from build123d import *

# Parameters (mm, degrees)
SKETCH_1_W             = 31
SKETCH_1_H             = 48
EXTRUDE_1_DEPTH        = 1.2
SKETCH_2_W             = 30.07
SKETCH_2_H             = 37.43
EXTRUDE_2_DEPTH        = 1.56
SKETCH_4_R             = 0.635
CUT_EXTRUDE_1_DEPTH    = 58.16146954
PATTERN_LINEAR_1_COUNT = 8
PATTERN_LINEAR_1_PITCH = 2.54
SKETCH_6_R             = 1
SKETCH_6_W             = 20
SKETCH_6_H             = 5.29
CUT_EXTRUDE_2_DEPTH    = 58.16146954


with BuildPart() as part:
    # 草图1 → 凸台-拉伸1 (new body)
    with BuildSketch(Plane(origin=(0, 0, 0), x_dir=(1, 0, 0), z_dir=(0, 1, 0))):
        with Locations((15.5, 24)):
            Rectangle(SKETCH_1_W, SKETCH_1_H)
    extrude(amount=EXTRUDE_1_DEPTH)

    # 草图2 → 凸台-拉伸2 (add)
    with BuildSketch(Plane(origin=(0, 1.2, 0), x_dir=(1, 0, 0), z_dir=(0, 1, 0))):
        with Locations((15.5, 24.005)):
            Rectangle(SKETCH_2_W, SKETCH_2_H)
    extrude(amount=EXTRUDE_2_DEPTH)

    # 草图4 → 切除-拉伸1 (cut, through all)
    with BuildSketch(Plane(origin=(0, 1.2, 0), x_dir=(1, 0, 0), z_dir=(0, 1, 0))):
        with Locations(Location((6.61, 46.5, 0), (0, 0, 270))):
            Circle(SKETCH_4_R)
    cut_extrude_1 = extrude(amount=-CUT_EXTRUDE_1_DEPTH, mode=Mode.SUBTRACT)

    # 阵列(线性)1: 切除-拉伸1 ×8
    with Locations(*[(i * PATTERN_LINEAR_1_PITCH, 0, 0) for i in range(1, PATTERN_LINEAR_1_COUNT)]):
        add(cut_extrude_1, mode=Mode.SUBTRACT)

    # 草图6 → 切除-拉伸2 (cut, through all)
    with BuildSketch(Plane(origin=(0, 1.2, 0), x_dir=(1, 0, 0), z_dir=(0, 1, 0))):
        with Locations(Location((2.5, 45.5, 0), (0, 0, 270))):
            Circle(SKETCH_6_R)
        with Locations(Location((28.5, 45.5, 0), (0, 0, 270))):
            Circle(SKETCH_6_R)
        with Locations(Location((2.5, 2.5, 0), (0, 0, 270))):
            Circle(SKETCH_6_R)
        with Locations(Location((28.5, 2.5, 0), (0, 0, 270))):
            Circle(SKETCH_6_R)
        with Locations((15.5, 2.645)):
            Rectangle(SKETCH_6_W, SKETCH_6_H)
    extrude(amount=-CUT_EXTRUDE_2_DEPTH, mode=Mode.SUBTRACT)


solid = part.part
The model under review builds one solid part; all positions refer to its coordinate system, in mm. A direction names the side the tool comes from. Round coordinates to 2 decimals unless told otherwise and drop trailing zeros. Write each loop counter-clockwise with the first axis right and the second up, starting at its lowest first coordinate (ties: lowest second). Pieces come first, ordered by that corner, then holes. Notation, with made-up numbers: M 41,71.25 L 52,71.25 A7 cw 52,79.25 Z; hole C -10,-30.75 d11. An arc over 180 degrees is marked long. Use a Markdown table: item, result. Add a question column.
Q1. Machinability: for faces 4 (the face through (15, 2, -42.72)), 5 (the face through (29.49, 0.61, -2.63)), 6 (the face through (25.5, 1, -3)), which of the approach directions +Z, -Z, +X, -X, +Y, -Y give a long, thin tool a straight path to every point of the face, cutting with its end or side? Answer none if there is none.
Q2. Insertion check: pin 1 (0.8 mm diameter, centred on y = 2, z = -31.5, fed in from +X) (3 decimals); pin 2 (1.5 mm diameter, centred on x = 24.39, z = -46.5, fed in from +Y). Each pin has a flat end and moves straight along its axis. Give the tip position at first contact, or say it passes through.
Q3. We need section C-C, the plane x = 2.5. State the section outline as (y, z) points, plus the area to 3 significant figures.
Q4. To check wall thickness, follow line 1 (X direction, y = 0.6, z = -2.5); line 2 (X direction, y = 1.15, z = -3); line 3 (X direction, y = 2, z = -7.5) (3 decimals). State the ranges of each line that lie inside material, in increasing order.
Q5. We need section B-B, the plane y = 0.75. Count the separate pieces of the cut face and the enclosed holes in it, plus the area to 3 significant figures.
Q6. We need section A-A, the plane z = -2.5. State the section outline as (x, y) points, plus the area to 3 significant figures.
Q7. We need section D-D, the plane x = 21.85. State the section outline as (y, z) points (3 decimals), plus the area to 3 significant figures.
Q8. The part is to be moulded in two halves that separate along X. For faces 1 (the face through (3, 1, 0)), 2 (the face through (0, 1, -24)), 3 (the face through (22.041, 0.608, -45.894)), say which applies: pulls with the +X half, pulls with the -X half, needs draft (parallel to the pull), parting line crosses it, or undercut.
Findings below:
| question | item | result |
|---|---|---|
| 1 | face 4 | -Z, +X, -X, +Y |
| 1 | face 5 | +Y, -Y |
| 1 | face 6 | +Z, +Y, -Y |
| 2 | pin 1 | stops at x = 30.535 |
| 2 | pin 2 | stops at y = 1.2 |
| 3 | outline | M 0,-48 L 1.2,-48 L 1.2,-46.5 L 0,-46.5 Z; M 0,-44.5 L 1.2,-44.5 L 1.2,-42.72 L 2.76,-42.72 L 2.76,-5.29 L 1.2,-5.29 L 1.2,-3.5 L 0,-3.5 Z; M 0,-1.5 L 1.2,-1.5 L 1.2,0 L 0,0 Z |
| 3 | area | 111 mm² |
| 4 | line 1 | x = 0 to 1.5, 3.5 to 5.5, 25.5 to 27.5, 29.5 to 31 |
| 4 | line 2 | x = 0 to 1.63, 3.37 to 5.5, 25.5 to 27.63, 29.37 to 31 |
| 4 | line 3 | x = 0.465 to 30.535 |
| 5 | separate pieces | 1 |
| 5 | enclosed holes | 12 |
| 5 | area | 1,360 mm² |
| 6 | outline | M 0,0 L 1.5,0 L 1.5,1.2 L 0,1.2 Z; M 3.5,0 L 5.5,0 L 5.5,1.2 L 3.5,1.2 Z; M 25.5,0 L 27.5,0 L 27.5,1.2 L 25.5,1.2 Z; M 29.5,0 L 31,0 L 31,1.2 L 29.5,1.2 Z |
| 6 | area | 8.40 mm² |
| 7 | outline | M 0,-48 L 1.2,-48 L 1.2,-47.135 L 0,-47.135 Z; M 0,-45.865 L 1.2,-45.865 L 1.2,-42.72 L 2.76,-42.72 L 2.76,-5.29 L 0,-5.29 Z |
| 7 | area | 108 mm² |
| 8 | face 1 | needs draft |
| 8 | face 2 | pulls with the -X half |
| 8 | face 3 | undercut |
